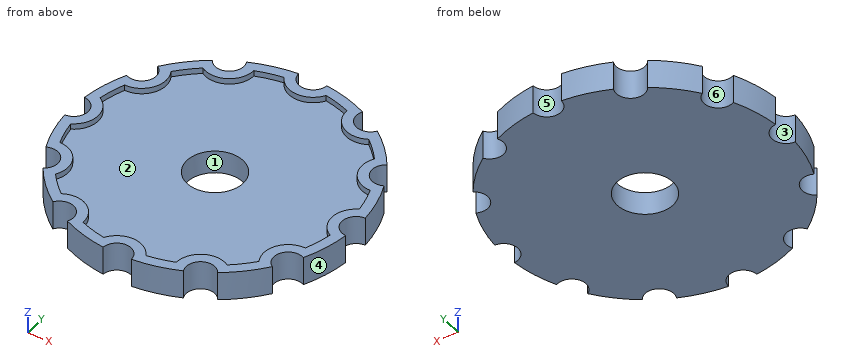
Autodesk Inventor part; units mm, degrees
ref_plane "YZ Plane" through (0, 0, 0) normal (1, 0, 0) x (0, 1, 0)
ref_plane "XZ Plane" through (0, 0, 0) normal (0, 1, 0) x (-1, 0, 0)
ref_plane "XY Plane" through (0, 0, 0) normal (0, 0, 1) x (1, 0, 0)
sketch "Sketch1" plane through (0, 0, 0) normal (0, 0, 1) x (1, 0, 0)
  circle A0 centre (0, 0) radius 12.7
  dimension "d9" = 25.4
extrude "Extrusion1" add sketch "Sketch1" along normal blind 2.54
sketch "Sketch2" plane through (0, 0, 2.54) normal (0, 0, 1) x (1, 0, 0)
  circle A0 centre (0, 12.7) radius 1.27
  dimension "d12" = 2.54
extrude "Extrusion2" cut sketch "Sketch2" against normal through all
pattern_circular "Circular Pattern1" count 12 over 360 about axis through (0, 0, 0) along (0, 0, 1) of "Extrusion2"
sketch "Sketch3" plane through (0, 0, 2.54) normal (0, 0, 1) x (1, 0, 0)
  arc A0 (5.2198, 11.5777) -> (7.4167, 10.3093) centre (6.35, 10.9985) ccw
  arc A1 (5.2198, 11.5777) -> (1.2684, 12.6365) centre (0, 0) ccw
  arc A2 (-1.2684, 12.6365) -> (1.2684, 12.6365) centre (0, 12.7) ccw
  arc A3 (-1.2684, 12.6365) -> (-5.2198, 11.5777) centre (0, 0) ccw
  arc A4 (-7.4167, 10.3093) -> (-5.2198, 11.5777) centre (-6.35, 10.9985) ccw
  arc A5 (-7.4167, 10.3093) -> (-10.3093, 7.4167) centre (0, 0) ccw
  arc A6 (-11.5777, 5.2198) -> (-10.3093, 7.4167) centre (-10.9985, 6.35) ccw
  arc A7 (-11.5777, 5.2198) -> (-12.6365, 1.2684) centre (0, 0) ccw
  arc A8 (-12.6365, -1.2684) -> (-12.6365, 1.2684) centre (-12.7, 0) ccw
  arc A9 (-12.6365, -1.2684) -> (-11.5777, -5.2198) centre (0, 0) ccw
  arc A10 (-10.3093, -7.4167) -> (-11.5777, -5.2198) centre (-10.9985, -6.35) ccw
  arc A11 (-10.3093, -7.4167) -> (-7.4167, -10.3093) centre (0, 0) ccw
  arc A12 (-5.2198, -11.5777) -> (-7.4167, -10.3093) centre (-6.35, -10.9985) ccw
  arc A13 (-5.2198, -11.5777) -> (-1.2684, -12.6365) centre (0, 0) ccw
  arc A14 (1.2684, -12.6365) -> (-1.2684, -12.6365) centre (0, -12.7) ccw
  arc A15 (1.2684, -12.6365) -> (5.2198, -11.5777) centre (0, 0) ccw
  arc A16 (7.4167, -10.3093) -> (5.2198, -11.5777) centre (6.35, -10.9985) ccw
  arc A17 (7.4167, -10.3093) -> (10.3093, -7.4167) centre (0, 0) ccw
  arc A18 (11.5777, -5.2198) -> (10.3093, -7.4167) centre (10.9985, -6.35) ccw
  arc A19 (11.5777, -5.2198) -> (12.6365, -1.2684) centre (0, 0) ccw
  arc A20 (12.6365, 1.2684) -> (12.6365, -1.2684) centre (12.7, 0) ccw
  arc A21 (12.6365, 1.2684) -> (11.5777, 5.2198) centre (0, 0) ccw
  arc A22 (10.3093, 7.4167) -> (11.5777, 5.2198) centre (10.9985, 6.35) ccw
  arc A23 (10.3093, 7.4167) -> (7.4167, 10.3093) centre (0, 0) ccw
  arc A24 (-1.8912, 11.6586) -> (-4.1914, 11.0423) centre (0, 0) ccw
  arc A25 (-1.8912, 11.6586) -> (1.8912, 11.6586) centre (0, 12.7) ccw
  arc A26 (4.1914, 11.0423) -> (1.8912, 11.6586) centre (0, 0) ccw
  arc A27 (4.1914, 11.0423) -> (7.4672, 9.151) centre (6.35, 10.9985) ccw
  arc A28 (9.151, 7.4672) -> (7.4672, 9.151) centre (0, 0) ccw
  arc A29 (9.151, 7.4672) -> (11.0423, 4.1914) centre (10.9985, 6.35) ccw
  arc A30 (11.6586, 1.8912) -> (11.0423, 4.1914) centre (0, 0) ccw
  arc A31 (11.6586, 1.8912) -> (11.6586, -1.8912) centre (12.7, 0) ccw
  arc A32 (11.0423, -4.1914) -> (11.6586, -1.8912) centre (0, 0) ccw
  arc A33 (11.0423, -4.1914) -> (9.151, -7.4672) centre (10.9985, -6.35) ccw
  arc A34 (7.4672, -9.151) -> (9.151, -7.4672) centre (0, 0) ccw
  arc A35 (7.4672, -9.151) -> (4.1914, -11.0423) centre (6.35, -10.9985) ccw
  arc A36 (1.8912, -11.6586) -> (4.1914, -11.0423) centre (0, 0) ccw
  arc A37 (1.8912, -11.6586) -> (-1.8912, -11.6586) centre (0, -12.7) ccw
  arc A38 (-4.1914, -11.0423) -> (-1.8912, -11.6586) centre (0, 0) ccw
  arc A39 (-4.1914, -11.0423) -> (-7.4672, -9.151) centre (-6.35, -10.9985) ccw
  arc A40 (-9.151, -7.4672) -> (-7.4672, -9.151) centre (0, 0) ccw
  arc A41 (-9.151, -7.4672) -> (-11.0423, -4.1914) centre (-10.9985, -6.35) ccw
  arc A42 (-11.6586, -1.8912) -> (-11.0423, -4.1914) centre (0, 0) ccw
  arc A43 (-11.6586, -1.8912) -> (-11.6586, 1.8912) centre (-12.7, 0) ccw
  arc A44 (-11.0423, 4.1914) -> (-11.6586, 1.8912) centre (0, 0) ccw
  arc A45 (-11.0423, 4.1914) -> (-9.151, 7.4672) centre (-10.9985, 6.35) ccw
  arc A46 (-7.4672, 9.151) -> (-9.151, 7.4672) centre (0, 0) ccw
  arc A47 (-7.4672, 9.151) -> (-4.1914, 11.0423) centre (-6.35, 10.9985) ccw
  dimension "d18" = 0.889
extrude "Extrusion3" cut sketch "Sketch3" against normal blind 0.508 contours A25 A26 A27 A28 A29 A30 A31 A32 A33 A34 A35 A36 A37 A38 A39 A40 A41 A42 A43 A44 A45 A46 A47 A24
hole "Hole1" at (0, 0, 0) direction (0, 0, 1) diameter 4.9784 end through all
properties part number "Tripod_Wheel" material "Polypropylene"
Can you work these out from the model? Positions are in its coordinate system, mm. Face numbers are marked on the shaded views. A direction names the side the tool comes from. Coordinates: 2 decimals unless noted, no trailing zeros. Write each loop counter-clockwise with the first axis right and the second up, starting at its lowest first coordinate (ties: lowest second). Pieces come first, ordered by that corner, then holes.
Q1. Please list where these lines run through material, in increasing order: L1, parallel to X at y = -10, z = 0.75; L2, parallel to Z at x = 8.25, y = -4.5.
Results found:
L1: x = -7.83 to -7.13, -5.57 to 5.57, 7.13 to 7.83
L2: z = 0 to 2.03
Q2. For P1, Ø1, axis at y = -8, z = 0.5, coming from the +X side; P2, Ø1, axis at y = 1.5, z = 1.5, coming from the -X side; P3, Ø4, axis at x = -7, y = -2.5, coming from the +Z side; P4, Ø1, axis at y = 0.5, z = 0.5, coming from the +X side, each with a flat end and sliding along its axis, tell me the tip position at first contact or that it passes through.
Results found:
P1: stops at x = 10.25
P2: stops at x = -12.64
P3: stops at z = 2.03
P4: stops at x = 11.92
Q3. Which directions (+Z, -Z, +X, -X, +Y, -Y) give clear straight access to the entire face, cutting with the end or side of a thin tool? Please do the marked faces 1 and 2.
Results found:
face 1: +Z, -Z
face 2: +Z
Q4. Imagine slicing it at B-B, the plane z = 0.4. List the corners of the cut face in (x, y) for me, plus the area to 3 significant figures.
Results found:
outline: (-12.64, -1.27) arc R12.7 ccw to (-11.58, -5.22) arc R1.27 cw to (-10.31, -7.42) arc R12.7 ccw to (-7.42, -10.31) arc R1.27 cw to (-5.22, -11.58) arc R12.7 ccw to (-1.27, -12.64) arc R1.27 cw to (1.27, -12.64) arc R12.7 ccw to (5.22, -11.58) arc R1.27 cw to (7.42, -10.31) arc R12.7 ccw to (10.31, -7.42) arc R1.27 cw to (11.58, -5.22) arc R12.7 ccw to (12.64, -1.27) arc R1.27 cw to (12.64, 1.27) arc R12.7 ccw to (11.58, 5.22) arc R1.27 cw to (10.31, 7.42) arc R12.7 ccw to (7.42, 10.31) arc R1.27 cw to (5.22, 11.58) arc R12.7 ccw to (1.27, 12.64) arc R1.27 cw to (-1.27, 12.64) arc R12.7 ccw to (-5.22, 11.58) arc R1.27 cw to (-7.42, 10.31) arc R12.7 ccw to (-10.31, 7.42) arc R1.27 cw to (-11.58, 5.22) arc R12.7 ccw to (-12.64, 1.27) arc R1.27 cw to start; hole circle Ø4.98 at (0, 0)
area: 457 mm2
Q5. If we mould it in two halves opening along X, with no side actions, what happens to the marked faces 3, 4, 5 and 6? For each: +X half, -X half, draft (parallel to the pull), parting line (faces both ways), or undercut.
Results found:
face 3: -X half
face 4: +X half
face 5: undercut
face 6: undercut
Q6. Imagine slicing it at C-C, the plane x = -6.35. List the corners of the cut face in (y, z) for me, plus the area to 3 significant figures.
Results found:
outline: (-9.73, 0) - (9.73, 0) - (9.73, 2.54) - (8.84, 2.54) - (8.84, 2.03) - (-8.84, 2.03) - (-8.84, 2.54) - (-9.73, 2.54) - close
area: 40.4 mm2
Q7. Imagine slicing it at A-A, the plane y = 0. List the corners of the cut face in (x, z) for me, plus the area to 3 significant figures.
Results found:
outline: (-11.43, 0) - (-2.49, 0) - (-2.49, 2.03) - (-10.54, 2.03) - (-10.54, 2.54) - (-11.43, 2.54) - close; (2.49, 0) - (11.43, 0) - (11.43, 2.54) - (10.54, 2.54) - (10.54, 2.03) - (2.49, 2.03) - close
area: 37.2 mm2
